Could you check a few things on this model? Use its own coordinates, in mm. Coordinates: 2 decimals unless noted, no trailing zeros. Loops run counter-clockwise (first coordinate to the right, second up) from the corner with the lowest first, then second, coordinate; pieces in that order, holes last.
Autodesk Inventor part; units mm, degrees
ref_plane "YZ Plane" through (0, 0, 0) normal (1, 0, 0) x (0, 1, 0)
ref_plane "XZ Plane" through (0, 0, 0) normal (0, 1, 0) x (-1, 0, 0)
ref_plane "XY Plane" through (0, 0, 0) normal (0, 0, 1) x (1, 0, 0)
sketch "Skizze2" plane through (0, 0, 0) normal (0, 0, 1) x (1, 0, 0)
  line L0 (-226.5, 226.5) -> (226.5, 226.5)
  line L1 (226.5, 226.5) -> (226.5, -226.5)
  line L2 (226.5, -226.5) -> (-226.5, -226.5)
  line L3 (-226.5, -226.5) -> (-226.5, 226.5)
  point P0 (0, 0)
  point P1 (0, 226.5)
  point P2 (-226.5, 0)
  dimension "d0" = 453
extrude "Extrusion1" add sketch "Skizze2" along normal blind 1
sketch "Skizze3" plane through (0, 0, 0) normal (0, 0, -1) x (-1, 0, 0)
  circle A0 centre (125, -208) radius 10
  line L0 (0, -317.1) -> (0, 317.1)
  line L1 (226.5, -226.5) -> (-226.5, -226.5)
  point P0 (0, 0)
  dimension "d3" = 20
  dimension "d4" = 125
  dimension "d5" = 18.5
extrude "Extrusion2" cut sketch "Skizze3" against normal blind 1
pattern_linear "Rechteckige Anordnung1" count 2 spacing 250 along (1, 0, 0) of "Extrusion2"
sketch "Skizze4" plane through (0, 0, 0) normal (0, 0, -1) x (-1, 0, 0)
  point P0 (0, 0)
  point P1 (160, -215)
  point P2 (-160, -215)
  point P3 (-160, 215)
  point P4 (160, 215)
  point P5 (0, 0)
  point P6 (-215, -145)
  point P7 (-215, 0)
  point P8 (-215, 145)
  point P9 (215, 145)
  point P10 (215, 0)
  point P11 (215, -145)
  point P12 (0, 0)
  point P13 (0, -145)
  point P14 (0, 145)
  dimension "d11" = 160
  dimension "d12" = 160
  dimension "d13" = 215
  dimension "d14" = 215
  dimension "d22" = 215
  dimension "d23" = 145
  dimension "d24" = 145
  dimension "d25" = 215
  dimension "d26" = 145
  dimension "d27" = 145
hole "Bohrung1" at (0, 0, 0) direction (0, 0, 1) diameter 3.4 depth 15 tip angle 118 countersink diameter 6.3 countersink angle 90
pattern_sketch "Skizzenbasierte Anordnung1" of "Bohrung1" from (0, 0, 0) copies at (-160, -215, 0) at (160, -215, 0) at (160, 215, 0) at (-160, 215, 0) at (215, -145, 0) at (215, 0, 0) at (215, 145, 0) at (-215, 145, 0) at (-215, 0, 0) at (-215, -145, 0) at (0, -145, 0) at (0, 145, 0)
equation "\"d10\" = 2 * d4"
properties part number "Rückplatte" material "PA 6.6"
(1) For pin 1 (18 mm diameter, centred on x = 125, y = -208, fed in from +Z), with a flat end and sliding along its axis, tell me the tip position at first contact or that it passes through.
Answers:
pin 1: passes through
(2) I need wall thicknesses on probe 1 along Y at (x, z) = (125, 0.4); probe 2 along Y at (x, z) = (161, 0.3); probe 3 along Y at (x, z) = (123, 0.15). Which ranges of each line are inside material? Lowest first, please.
Answers:
probe 1: y = -226.5 to -218, -198 to 226.5
probe 2: y = -226.5 to -217.67, -212.33 to 212.33, 217.67 to 226.5
probe 3: y = -226.5 to -217.8, -198.2 to 226.5
(3) We'd pull the mould along Y, two halves only. Please class faces 1 (the face through (-122.83, -217.76, 0.49)), 2 (the face through (-3, 3, 1)): +Y half, -Y half, draft (parallel to the pull), parting line (faces both ways), or undercut.
Answers:
face 1: undercut
face 2: draft
(4) Imagine slicing it at A-A, the plane x = 125. Write out the boundary of the cut face in (y, z), and give its area (3 significant figures).
Answers:
outline: (-226.5, 0) - (-218, 0) - (-218, 1) - (-226.5, 1) - close; (-198, 0) - (226.5, 0) - (226.5, 1) - (-198, 1) - close
area: 433 mm2
